```python
from build123d import *

# Parameters (mm, degrees)
SKETCH1_R           = 2.5
BOSS_EXTRUDE1_DEPTH = 0.6
FILLET1_R           = 0.2


with BuildPart() as part:
    # Sketch1 → Boss-Extrude1 (new body)
    with BuildSketch(Plane(origin=(0, 0, 0), x_dir=(1, 0, 0), z_dir=(0, 1, 0))):
        with Locations(Location((0, 0, 0), (0, 0, 270))):
            Circle(SKETCH1_R)
    extrude(amount=BOSS_EXTRUDE1_DEPTH)

    # Loft1: read off the stored shape, not the designer's step
    # Loft1: loft between two sections, ruled curve by curve
    loft1_from = [
        Edge.make_bspline([(-0.886625195, 0.6, 2.337497757), (3.788370319, 0.6, 4.110748147), (5.561620709, 0.6, -0.564247367), (0.886625195, 0.6, -2.337497757), (-3.788370319, 0.6, -4.110748147), (-5.561620709, 0.6, 0.564247367), (-0.886625195, 0.6, 2.337497757)], [0, 0, 0, 0, 0.5, 0.5, 0.5, 1, 1, 1, 1], 3, [1, 0.333333333, 0.333333333, 1, 0.333333333, 0.333333333, 1]),
    ]
    loft1_to = [
        Edge.make_bspline([(0.573645482, 5.6, 4.966984081), (10.507613644, 5.6, 3.819693116), (9.36032268, 5.6, -6.114275046), (-0.573645482, 5.6, -4.966984081), (-10.507613644, 5.6, -3.819693116), (-9.36032268, 5.6, 6.114275046), (0.573645482, 5.6, 4.966984081)], [0, 0, 0, 0, 0.5, 0.5, 0.5, 1, 1, 1, 1], 3, [1, 0.333333333, 0.333333333, 1, 0.333333333, 0.333333333, 1]),
    ]
    loft1 = Solid(Shell([*[Face.make_surface_from_curves(loft1_from[k], loft1_to[k]) for k in range(1)], Face(Wire(loft1_from)), Face(Wire(loft1_to))]))
    add(loft1)

    # Fillet1
    fillet1_edges = [part.edges().sort_by_distance(p)[0] for p in [
        (-0.573645482, 5.6, -4.966984081),
    ]]
    fillet(fillet1_edges, radius=FILLET1_R)


solid = part.part
```
Design review of the part built by this model. Coordinates are the model's own, in mm. A direction names the side the tool comes from. Give positions to 0.01 mm unless a question says otherwise; leave off trailing zeros. Use a Markdown table: item, result. Add a question column.
(1) Machinability: for faces 1 (the face through (-2.44, 0.3, -0.54)), 2 (the face through (0, 0, 0)), which of the approach directions +Z, -Z, +X, -X, +Y, -Y give a long, thin tool a straight path to every point of the face, cutting with its end or side? Answer none if there is none.
(2) Clearance check with flat-ended pins moving along their axes: P1, Ø1, axis at x = -2, z = -1.5, coming from the -Y side; P2, Ø3, axis at x = -3, y = 1.5, coming from the -Z side; P3, Ø2, axis at x = -4, y = 4, coming from the +Z side. State where each tip first meets the part, or that it passes through.
(3) Wall thickness on probe 1 along X at (y, z) = (0.6, 0); probe 2 along Z at (x, y) = (3.75, 4.1); probe 3 along Z at (x, y) = (3.75, 4.9): over which ranges is each line inside the solid? List them lowest first. Write a range as [from, to].
Report:
| question | item | result |
|---|---|---|
| 1 | face 1 | -Y |
| 1 | face 2 | +Z, -Z, +X, -X, -Y |
| 2 | P1 | stops at y = 0 |
| 2 | P2 | stops at z = -2.78 |
| 2 | P3 | stops at z = 3.09 |
| 3 | probe 1 | x = [-2.5, 2.5] |
| 3 | probe 2 | z = [-1.85, 1.85] |
| 3 | probe 3 | z = [-2.69, 2.69] |
